Autodesk Inventor part; units mm, degrees
ref_plane "YZ Plane" through (0, 0, 0) normal (1, 0, 0) x (0, 1, 0)
ref_plane "XZ Plane" through (0, 0, 0) normal (0, 1, 0) x (-1, 0, 0)
ref_plane "XY Plane" through (0, 0, 0) normal (0, 0, 1) x (1, 0, 0)
sketch "Sketch1" plane through (0, 0, 0) normal (0, 0, 1) x (1, 0, 0)
  arc A0 (-1.5748, -2.3876) -> (-1.5748, 2.3876) centre (-1.5748, 0) ccw
  line L0 (-1.5748, 2.3876) -> (-3.1623, 2.3876)
  line L1 (-1.5748, -2.3876) -> (-3.1623, -2.3876)
  line L2 (2.286, -2.54) -> (2.286, 2.54)
  line L3 (2.286, 2.54) -> (3.0412, 2.54)
  line L4 (2.286, -2.54) -> (3.0412, -2.54)
  arc A1 (-3.1623, -2.3876) -> (3.0412, -2.54) centre (0, 0) ccw
  arc A2 (3.0412, 2.54) -> (-3.1623, 2.3876) centre (0, 0) ccw
  point P0 (2.286, 0)
  dimension "d2" = 1.5748
  dimension "d3" = 5.08
  dimension "d4" = 2.286
  dimension "d5" = 3.9624
  dimension "d13" = 3.9624
  dimension "d14" = 0.1524
  dimension "d15" = 2.3876
extrude "Extrusion1" add sketch "Sketch1" along normal blind 787.4
sketch "Sketch2" plane through (0, 0, 787.4) normal (0, 0, 1) x (1, 0, 0)
  arc A0 (-1.5748, -2.3876) -> (-1.5748, 2.3876) centre (-1.5748, 0) ccw
  line L0 (-1.5748, -2.3876) -> (-3.1623, -2.3876)
  arc A1 (-3.1623, -2.3876) -> (3.0412, -2.54) centre (0, 0) ccw
  line L1 (3.0412, -2.54) -> (2.286, -2.54)
  line L2 (2.286, -2.54) -> (2.286, 2.54)
  line L3 (2.286, 2.54) -> (3.0412, 2.54)
  arc A2 (3.0412, 2.54) -> (-3.1623, 2.3876) centre (0, 0) ccw
  line L4 (-3.1623, 2.3876) -> (-1.5748, 2.3876)
sketch "Sketch3" plane through (0, 0, 787.4) normal (0, 0, 1) x (1, 0, 0)
  arc A0 (-1.5748, -2.3876) -> (-1.5748, 2.3876) centre (-1.5748, 0) ccw
  line L0 (-1.5748, -2.3876) -> (-3.1623, -2.3876)
  arc A1 (-3.1623, -2.3876) -> (3.0412, -2.54) centre (0, 0) ccw
  line L1 (3.0412, -2.54) -> (2.286, -2.54)
  line L2 (2.286, -2.54) -> (2.286, 2.54)
  line L3 (2.286, 2.54) -> (3.0412, 2.54)
  arc A2 (3.0412, 2.54) -> (-3.1623, 2.3876) centre (0, 0) ccw
  line L4 (-3.1623, 2.3876) -> (-1.5748, 2.3876)
sketch "Sketch4" plane through (0, 0, 787.4) normal (0, 0, 1) x (1, 0, 0)
  arc A0 (-1.5748, -2.3876) -> (-1.5748, 2.3876) centre (-1.5748, 0) ccw
  line L0 (-1.5748, -2.3876) -> (-3.1623, -2.3876)
  arc A1 (-3.1623, -2.3876) -> (3.0412, -2.54) centre (0, 0) ccw
  line L1 (3.0412, -2.54) -> (2.286, -2.54)
  line L2 (2.286, -2.54) -> (2.286, 2.54)
  line L3 (2.286, 2.54) -> (3.0412, 2.54)
  arc A2 (3.0412, 2.54) -> (-3.1623, 2.3876) centre (0, 0) ccw
  line L4 (-3.1623, 2.3876) -> (-1.5748, 2.3876)
properties part number "thin rod" material "Polyethylene, High Density"
Could you check a few things on this model? Use its own coordinates, in mm. Round coordinates to 2 decimals unless told otherwise and drop trailing zeros. Write each loop counter-clockwise with the first axis right and the second up, starting at its lowest first coordinate (ties: lowest second). Pieces come first, ordered by that corner, then holes. Notation, with made-up numbers: M 78,78 L 117,78 A32 cw 117,113 Z; hole C 75,45 d2. An arc over 180 degrees is marked long. Answer in a Markdown table with one row per item. Add a question column.
Q1. Imagine slicing it at B-B (y = 0). Please give me the cut outline in (x, z).
Q2. If I drill on line 1 (Y direction, x = 1, z = 667); line 2 (Y direction, x = -0.5, z = 223); line 3 (Y direction, x = 2.5, z = 330.5), over which ranges is the centre line in solid material (lowest first)? Write a range as from..to.
Q3. Will these pins go through, and if not, where does the flat tip stop? pin 1 Ø1.7 at (x, z) = (-2.5, 374) entering from +Y; pin 2 Ø3 at (y, z) = (0, 501) entering from -X; pin 3 Ø0.5 at (x, z) = (-2.5, 263) entering from -Y; pin 4 Ø2 at (x, y) = (-1, -1) entering from +Z.
Q4. Imagine slicing it at A-A (z = 651). Please give me the cut outline in (x, y).
Values:
| question | item | result |
|---|---|---|
| 1 | outline | M 0.81,0 L 2.29,0 L 2.29,787.4 L 0.81,787.4 Z |
| 2 | line 1 | -3.83..3.83 |
| 2 | line 2 | -3.93..-2.13, 2.13..3.93 |
| 2 | line 3 | -3.07..-2.54, 2.54..3.07 |
| 3 | pin 1 | y = 3.6 |
| 3 | pin 2 | x = 0.28 |
| 3 | pin 3 | y = -3.26 |
| 3 | pin 4 | through |
| 4 | outline | M -3.16,-2.39 A3.96 ccw 3.04,-2.54 L 2.29,-2.54 L 2.29,2.54 L 3.04,2.54 A3.96 ccw -3.16,2.39 L -1.57,2.39 A2.39 cw -1.57,-2.39 Z |
